Here's how the part is built. I have some questions about the finished solid (model axes, mm). A direction names the side the tool comes from. Give positions to 0.01 mm unless a question says otherwise; leave off trailing zeros. Loops run counter-clockwise (first coordinate to the right, second up) from the corner with the lowest first, then second, coordinate; pieces in that order, holes last.
Q1. We'd pull the mould along X, two halves only. Please class faces 3 (the face through (1.75, -9.41, 5.11)), 4 (the face through (-2.17, -9.76, 9.71)), 5 (the face through (1.697, 9.397, 3.853)), 6 (the face through (0, 0, 0)): +X half, -X half, draft (parallel to the pull), parting line (faces both ways), or undercut.
Q2. Will these pins go through, and if not, where does the flat tip stop? P1, Ø12, axis at x = -0.5, y = -4.5, coming from the +Z side; P2, Ø11, axis at x = 0, y = 0, coming from the +Z side; P3, Ø4, axis at x = 3.5, z = 6, coming from the -Y side; P4, Ø2, axis at x = -3.5, z = 4.5, coming from the -Y side.
Q3. I need wall thicknesses on line 1 (Y direction, x = 0, z = 9.5); line 2 (Z direction, x = 0, y = -9.65); line 3 (Z direction, x = -5, y = -2.25). Which ranges of each line are inside material? Lowest first, please.
Q4. If we section it at B-B (y = 0): Please give me the cut outline in (x, z), plus the area to 3 significant figures.
Q5. If we section it at A-A (x = 0): Please give me the cut outline in (y, z), plus the area to 3 significant figures.
Q6. If we section it at C-C (z = 15.25): Please give me the cut outline in (x, y), plus the area to 3 significant figures.
Q7. For faces 1 (the face through (-9, 2, 19.7)), 2 (the face through (-1.951, -8.786, 10.219)), which set-ups out of +Z, -Z, +X, -X, +Y, -Y let a thin tool reach every point of the face, with its end or its side?
Q8. If we section it at D-D (x = 7.75): Please give me the cut outline in (y, z), plus the area to 3 significant figures.
from build123d import *

# Parameters (mm, degrees)
F0_R     = 10
F1_DEPTH = 19.7
F2_T     = -1
F3_R     = 1.837004
F4_DEPTH = 11.6


with BuildPart() as f1:
    # F0 (on Top) → F1 (new body)
    with BuildSketch(Plane.XY):
        Circle(F0_R)
    extrude(amount=F1_DEPTH)

    # F2
    f2_openings = [f1.faces().sort_by_distance(p)[0] for p in [
        (0, 0, 19.7),
    ]]
    offset(amount=F2_T, openings=f2_openings)

    # F3 (on Front) → F4 (cut, symmetric)
    with BuildSketch(Plane.XZ):
        with Locations((0, 4.556882)):
            Circle(F3_R)
    extrude(amount=F4_DEPTH, both=True, mode=Mode.SUBTRACT)


solid = f1.part
Check sheet entries:
1. face 3: undercut
1. face 4: parting line
1. face 5: undercut
1. face 6: draft
2. P1: stops at z = 19.7
2. P2: stops at z = 1
2. P3: stops at y = -9.89
2. P4: stops at y = -9.68
3. line 1: y = -10 to -9, 9 to 10
3. line 2: z = 0 to 2.72, 6.39 to 19.7
3. line 3: z = 0 to 1
4. outline: (-10, 0) - (10, 0) - (10, 19.7) - (9, 19.7) - (9, 1) - (-9, 1) - (-9, 19.7) - (-10, 19.7) - close
4. area: 57.4 mm2
5. outline: (-10, 0) - (10, 0) - (10, 2.72) - (9, 2.72) - (9, 1) - (-9, 1) - (-9, 2.72) - (-10, 2.72) - close; (-10, 6.39) - (-9, 6.39) - (-9, 19.7) - (-10, 19.7) - close; (9, 6.39) - (10, 6.39) - (10, 19.7) - (9, 19.7) - close
5. area: 50.1 mm2
6. outline: circle Ø20 at (0, 0); hole circle Ø18 at (0, 0)
6. area: 59.7 mm2
7. face 1: +Z, +X, -X, +Y, -Y
7. face 2: +Z
8. outline: (-6.32, 0) - (6.32, 0) - (6.32, 19.7) - (4.58, 19.7) - (4.58, 1) - (-4.58, 1) - (-4.58, 19.7) - (-6.32, 19.7) - close
8. area: 77.9 mm2
